Design review of the part built by this model. Coordinates are the model's own, in mm. A direction names the side the tool comes from. Coordinates: 2 decimals unless noted, no trailing zeros. Loops run counter-clockwise (first coordinate to the right, second up) from the corner with the lowest first, then second, coordinate; pieces in that order, holes last. Notation, with made-up numbers: (1, 88) - (24, 88) arc R16 cw to (24, 92) - close; hole circle Ø6 at (49, 46). An arc over 180 degrees is marked (long way). One line per question, with ' | ' between items.
Autodesk Inventor part; units mm, degrees
ref_plane "YZ Plane" through (0, 0, 0) normal (1, 0, 0) x (0, 1, 0)
ref_plane "XZ Plane" through (0, 0, 0) normal (0, 1, 0) x (-1, 0, 0)
ref_plane "XY Plane" through (0, 0, 0) normal (0, 0, 1) x (1, 0, 0)
sketch "スケッチ5" plane through (0, 0, 3.2) normal (0, 0, 1) x (1, 0, 0)
  circle A0 centre (-16.1762, 60.3704) radius 1.621
  circle A1 centre (16.1762, 60.3704) radius 1.621
  arc A2 (67.5, 0) -> (-67.5, 0) centre (0, 0) ccw
  circle A3 centre (-16.1762, 60.3704) radius 5
  circle A4 centre (16.1762, 60.3704) radius 5
  circle A5 centre (-44.1942, 44.1942) radius 1.621
  circle A6 centre (-60.3704, 16.1762) radius 1.621
  circle A7 centre (44.1942, 44.1942) radius 1.621
  circle A8 centre (60.3704, 16.1762) radius 1.621
  arc A9 (62.5, 0) -> (-62.5, 0) centre (0, 0) ccw
  circle A10 centre (-44.1942, 44.1942) radius 5
  circle A11 centre (-60.3704, 16.1762) radius 5
  circle A12 centre (44.1942, 44.1942) radius 5
  circle A13 centre (60.3704, 16.1762) radius 5
  line L0 (-45.5, 0) -> (-67.5, 0)
  line L1 (67.5, 0) -> (45.5, 0)
  point P0 (17.4703, 65.2)
  point P1 (-17.4703, 65.2)
  point P2 (58.8841, 20.9502)
  point P3 (65.2, 17.4703)
  point P4 (47.7297, 47.7297)
  point P5 (47.5855, 40.52)
  point P6 (40.52, 47.5855)
  point P7 (20.9502, 58.8841)
  point P8 (-65.2, 17.4703)
  point P9 (-58.8841, 20.9502)
  point P10 (-47.5855, 40.52)
  point P11 (-47.7297, 47.7297)
  point P12 (-40.52, 47.5855)
  point P13 (-20.9502, 58.8841)
  point P14 (-11.2987, 61.4702)
  point P15 (11.2987, 61.4702)
  point P16 (61.4702, 11.2987)
  point P17 (-61.4702, 11.2987)
sketch "スケッチ1" plane through (0, 0, 0) normal (0, 0, 1) x (1, 0, 0)
  arc A0 (45.5, 0) -> (-45.5, 0) centre (0, 0) ccw
  arc A1 (67.5, 0) -> (-67.5, 0) centre (0, 0) ccw
  line L0 (-44.5, 0) -> (0, 0)
  line L1 (-67.5, 0) -> (67.5, 0)
  dimension "d0" = 91
  dimension "d1" = 135
  dimension "d5" = 0
extrude "プレート2" add sketch "スケッチ1" along normal blind 3.2 contours A0 L1 A1
sketch "スケッチ2" plane through (0, 0, 3.2) normal (0, 0, 1) x (1, 0, 0)
  circle A0 centre (0, 0) radius 62.5
  point P0 (16.1762, 60.3704)
  point P1 (-16.1762, 60.3704)
  point P2 (-44.1942, 44.1942)
  point P3 (-60.3704, 16.1762)
  point P4 (-60.3704, -16.1762)
  point P5 (-44.1942, -44.1942)
  point P6 (-16.1762, -60.3704)
  point P7 (16.1762, -60.3704)
  point P8 (44.1942, -44.1942)
  point P9 (60.3704, -16.1762)
  point P10 (60.3704, 16.1762)
  point P11 (44.1942, 44.1942)
  dimension "d8" = 125
  dimension "d11" = 360
  dimension "d49" = 0
hole "穴1" at (16.1762, 60.3704, 3.2) at (-16.1762, 60.3704, 3.2) at (-44.1942, 44.1942, 3.2) at (-60.3704, 16.1762, 3.2) at (-60.3704, -16.1762, 3.2) at (-44.1942, -44.1942, 3.2) at (-16.1762, -60.3704, 3.2) at (16.1762, -60.3704, 3.2) at (44.1942, -44.1942, 3.2) at (60.3704, -16.1762, 3.2) at (60.3704, 16.1762, 3.2) at (44.1942, 44.1942, 3.2) direction (0, 0, -1) diameter 3.242 end through all
sketch "スケッチ6" plane through (0, 0, 3.2) normal (0, 0, 1) x (1, 0, 0)
  arc A0 (45.5, 0) -> (-45.5, 0) centre (0, 0) ccw
  line L0 (-32.1734, 32.1734) -> (0, 0)
  line L1 (0, 0) -> (32.1734, 32.1734)
  line L2 (0, 81) -> (0, -13.5)
  arc A1 (41.5, 0) -> (-41.5, 0) centre (0, 0) ccw
  point P0 (-29.3449, 29.3449)
  point P1 (29.3449, 29.3449)
  dimension "d50" = 45
  dimension "d51" = 45
  dimension "d56" = 4
extrude "押し出し2" add sketch "スケッチ6" against normal up to surface (3.2 mm away) contours L1 A1 L2 A0 | L2 A1 L0 A0
fillet "コーナーR7" radius 1 4 edges at (-29.3449, 29.3449, 1.6) (29.3449, 29.3449, 1.6) (-32.1734, 32.1734, 1.6) (32.1734, 32.1734, 1.6)
equation "\"d18\" = Thickness"
equation "\"d6\" = Thickness"
equation "\"BendRadius\" = Thickness"
equation "\"BendReliefWidth\" = Thickness"
equation "\"BendReliefDepth\" = 0.5 * Thickness"
equation "\"CornerReliefSize\" = 4 * Thickness"
equation "\"MinimumRemnant\" = 2 * Thickness"
equation "\"TransitionRadius\" = BendRadius"
equation "\"JacobiRadiusSize\" = BendRadius"
equation "\"GapSize\" = Thickness"
properties part number "plate1" material "鋼、炭素鋼"
Q1. Take a section at A-A (y = 20.5). Give the boundary of the cut face in (x, z).
Returned:
outline: (-64.31, 0) - (-40.62, 0) - (-40.62, 3.2) - (-64.31, 3.2) - close; (40.62, 0) - (64.31, 0) - (64.31, 3.2) - (40.62, 3.2) - close
Q2. Take a section at D-D (y = 53). Give the boundary of the cut face in (x, z).
Returned:
outline: (-41.8, 0) - (41.8, 0) - (41.8, 3.2) - (-41.8, 3.2) - close
Q3. Tool access review of faces 1 (the cylindrical face through (42.14, 17.16, 1.58)), 2 (the flat face through (56, 0, 2)): name each direction out of +Z, -Z, +X, -X, +Y, -Y from which nothing blocks a thin tool from reaching the whole face with its end or side.
Returned:
face 1: +Z, -Z, -Y | face 2: +Z, -Z, +X, -X, -Y
Q4. For pin 1 (1.9 mm diameter, centred on x = -60.37, y = 16.18, fed in from +Z), flat-tipped, find the tip position at first contact; note if it passes through.
Returned:
pin 1: passes through
Q5. To check wall thickness, follow line 1 along X through (y, z) = (60.5, 1.3); line 2 along X through (y, z) = (61, 2.4); line 3 along X through (y, z) = (17.5, 1.1). State the ranges of each line that lie inside material, in increasing order.
Returned:
line 1: x = -29.93 to -17.79, -14.56 to 14.56, 17.79 to 29.93 | line 2: x = -28.9 to -17.67, -14.68 to 14.68, 17.67 to 28.9 | line 3: x = -65.19 to -61.31, -59.43 to -42, 42 to 59.43, 61.31 to 65.19
Q6. Take a section at C-C (z = 2.35). Give the boundary of the cut face in (x, y), plus the area to 3 significant figures.
Returned:
outline: (-67.5, 0) - (-45.5, 0) arc R45.5 cw to (-32.89, 31.44) arc R1 cw to (-31.46, 31.46) - (-30.04, 30.04) arc R1 ccw to (-28.65, 30.03) arc R41.5 cw to (28.65, 30.03) arc R1 ccw to (30.04, 30.04) - (31.46, 31.46) arc R1 cw to (32.89, 31.44) arc R45.5 cw to (45.5, 0) - (67.5, 0) arc R67.5 ccw to start; hole circle Ø3.24 at (-60.37, 16.18); hole circle Ø3.24 at (-44.19, 44.19); hole circle Ø3.24 at (-16.18, 60.37); hole circle Ø3.24 at (16.18, 60.37); hole circle Ø3.24 at (44.19, 44.19); hole circle Ø3.24 at (60.37, 16.18) | area: 4,130 mm²
Q7. Draft analysis for pull direction Y (two halves, no side actions). For faces 3 (the cylindrical face through (60.99, 14.68, 1.58)), 4 (the cylindrical face through (0.4, 41.5, 1.6)), 5 (the cylindrical face through (-1.484, 67.484, 1.578)), 6 (the cylindrical face through (-61.737, 15.305, 1.578)), state which applies: +Y half, -Y half, draft (parallel to the pull), parting line (faces both ways), or undercut.
Returned:
face 3: undercut | face 4: -Y half | face 5: +Y half | face 6: undercut
Q8. Take a section at B-B (x = 0). Give the boundary of the cut face in (y, z).
Returned:
outline: (41.5, 0) - (67.5, 0) - (67.5, 3.2) - (41.5, 3.2) - close
